from build123d import *

# Parameters (mm, degrees)
BOSS_EXTRUDE1_DEPTH = 3.175


with BuildPart() as part:
    # Sketch2 → Boss-Extrude1 (new body)
    with BuildSketch(Plane.XY):
        with BuildLine():
            Line((-1, 10), (104, 10))
            ThreePointArc((104, 10), (107.535533906, 8.535533906), (109, 5))
            Line((109, 5), (109, -83.5))
            ThreePointArc((109, -83.5), (107.535533906, -87.035533906), (104, -88.5))
            Line((104, -88.5), (-1, -88.5))
            ThreePointArc((-1, -88.5), (-4.535533906, -87.035533906), (-6, -83.5))
            Line((-6, -83.5), (-6, 5))
            ThreePointArc((-6, 5), (-4.535533906, 8.535533906), (-1, 10))
        make_face()
        with BuildLine():
            Line((5.5, 0), (5.5, -1))
            ThreePointArc((5.5, -1), (5.353553391, -1.353553391), (5, -1.5))
            Line((5, -1.5), (3, -1.5))
            ThreePointArc((3, -1.5), (1.5, -3), (3, -4.5))
            Line((3, -4.5), (5, -4.5))
            ThreePointArc((5, -4.5), (5.353553391, -4.646446609), (5.5, -5))
            Line((5.5, -5), (5.5, -73.5))
            ThreePointArc((5.5, -73.5), (5.353553391, -73.853553391), (5, -74))
            Line((5, -74), (3, -74))
            ThreePointArc((3, -74), (1.5, -75.5), (3, -77))
            Line((3, -77), (5, -77))
            ThreePointArc((5, -77), (5.353553391, -77.146446609), (5.5, -77.5))
            Line((5.5, -77.5), (5.5, -78.5))
            Line((5.5, -78.5), (96.149180328, -78.5))
            Line((96.149180328, -78.5), (96.149180328, -77.5))
            ThreePointArc((96.149180328, -77.5), (96.295626937, -77.146446609), (96.649180328, -77))
            Line((96.649180328, -77), (98.649180328, -77))
            ThreePointArc((98.649180328, -77), (100.149180328, -75.5), (98.649180328, -74))
            Line((98.649180328, -74), (96.649180328, -74))
            ThreePointArc((96.649180328, -74), (96.295626937, -73.853553391), (96.149180328, -73.5))
            Line((96.149180328, -73.5), (96.149180328, -5))
            ThreePointArc((96.149180328, -5), (96.295626937, -4.646446609), (96.649180328, -4.5))
            Line((96.649180328, -4.5), (98.649180328, -4.5))
            ThreePointArc((98.649180328, -4.5), (100.149180328, -3), (98.649180328, -1.5))
            Line((98.649180328, -1.5), (96.649180328, -1.5))
            ThreePointArc((96.649180328, -1.5), (96.295626937, -1.353553391), (96.149180328, -1))
            Line((96.149180328, -1), (96.149180328, 0))
            Line((96.149180328, 0), (5.5, 0))
        make_face(mode=Mode.SUBTRACT)
    extrude(amount=BOSS_EXTRUDE1_DEPTH)


solid = part.part
Verification items for the finished model (mm, model axes). A direction names the side the tool comes from. Coordinates: 2 decimals unless noted, no trailing zeros. Write each loop counter-clockwise with the first axis right and the second up, starting at its lowest first coordinate (ties: lowest second). Pieces come first, ordered by that corner, then holes. Notation, with made-up numbers: (75, 44.25) - (115, 44.25) arc R17 ccw to (115, 57.25) - close; hole circle Ø5 at (35, -36). An arc over 180 degrees is marked (long way). Answer as a JSON object with one key per item and string values.
(1) Cross-section at A-A on y = -3. Record the cut outline in (x, z) (3 decimals), plus the area to 3 significant figures.
Report:
{"outline": "(-6, 0) - (1.5, 0) - (1.5, 3.175) - (-6, 3.175) - close; (100.149, 0) - (109, 0) - (109, 3.175) - (100.149, 3.175) - close", "area": "51.9 mm^2"}
(2) Thickness scan on line 1 along Y through (x, z) = (66.5, 2.6); line 2 along X through (y, z) = (-57, 1.8); line 3 along X through (y, z) = (-76.5, 1.55). Record the ranges inside material, lowest first.
Report:
{"line 1": "-88.5 to -78.5, 0 to 10", "line 2": "-6 to 5.5, 96.15 to 109", "line 3": "-6 to 1.88, 99.77 to 109"}
(3) Cross-section at B-B on x = 22. Record the cut outline in (y, z) (3 decimals).
Report:
{"outline": "(-88.5, 0) - (-78.5, 0) - (-78.5, 3.175) - (-88.5, 3.175) - close; (0, 0) - (10, 0) - (10, 3.175) - (0, 3.175) - close"}
(4) Tool access check on faces 1 (the flat face through (50, -78.5, 2)), 2 (the flat face through (51, 10, 2)). Record the directions out of +Z, -Z, +X, -X, +Y, -Y that give a thin tool (end or side, any length) a straight path to the whole face; none if there is none.
Report:
{"face 1": "+Z, -Z", "face 2": "+Z, -Z, +X, -X, +Y"}
(5) Mould release check, pull along Y, two halves, no side actions. Record for faces 3 (the flat face through (52, -88.5, 2)), 4 (the flat face through (109, -39, 2)), 5 (the cylindrical face through (100.15, -75.53, 1.57)): pulls with the +Y half, pulls with the -Y half, needs draft (parallel to the pull), parting line crosses it, or undercut.
Report:
{"face 3": "pulls with the -Y half", "face 4": "needs draft", "face 5": "undercut"}
